Can you work these out from the model? Positions are in its coordinate system, mm. A direction names the side the tool comes from. Give positions to 0.01 mm unless a question says otherwise; leave off trailing zeros. Loops run counter-clockwise (first coordinate to the right, second up) from the corner with the lowest first, then second, coordinate; pieces in that order, holes last. Notation, with made-up numbers: (21, 51.5) - (57, 51.5) arc R33 ccw to (57, 83.5) - close; hole circle Ø4 at (4.25, 76.25). An arc over 180 degrees is marked (long way). Answer in a Markdown table with one row per item.
from build123d import *

# Parameters (mm, degrees)
SKETCH1_R           = 2
BOSS_EXTRUDE1_DEPTH = 75


# Read off the part's stored shape, not the designer's step: M5 Tapped Hole1
with BuildPart() as part:
    # Sketch1 → Boss-Extrude1 (new, symmetric)
    with BuildSketch(Plane(origin=(0, 0, 0), x_dir=(0, 0, -1), z_dir=(1, 0, 0))):
        with BuildLine():
            Line((-10, 0), (-8.2, 0))
            Line((-8.2, 0), (-8.2, -2.5))
            Line((-8.2, -2.5), (-6.43933983, -2.5))
            Line((-6.43933983, -2.5), (-2.839339831, -6.099999999))
            Line((-2.839339831, -6.099999999), (2.839339828, -6.099999999))
            Line((2.839339828, -6.099999999), (6.439339829, -2.499999999))
            Line((6.439339829, -2.499999999), (8.2, -2.499999999))
            Line((8.2, -2.499999999), (8.2, 0))
            Line((8.2, 0), (10, 0))
            Line((10, 0), (10, -5.167329724))
            ThreePointArc((10, -5.167329724), (9.953566515, -5.400766617), (9.821335137, -5.59866486))
            Line((9.821335137, -5.59866486), (8.541421356, -6.87857864))
            ThreePointArc((8.541421356, -6.87857864), (8.323463314, -6.921933191), (8.2, -6.737157284))
            Line((8.2, -6.737157284), (8.2, -3.999999998))
            Line((8.2, -3.999999998), (7.06066017, -3.999999998))
            Line((7.06066017, -3.999999998), (3.9, -7.160660168))
            Line((3.9, -7.160660168), (3.9, -12.83933983))
            Line((3.9, -12.83933983), (6.560660169, -15.499999999))
            Line((6.560660169, -15.499999999), (8.2, -15.499999999))
            Line((8.2, -15.499999999), (8.2, -13.262842712))
            ThreePointArc((8.2, -13.262842712), (8.323463314, -13.078066805), (8.541421356, -13.121421355))
            Line((8.541421356, -13.121421355), (9.821335137, -14.401335136))
            ThreePointArc((9.821335137, -14.401335136), (9.953566515, -14.599233379), (10, -14.832670272))
            Line((10, -14.832670272), (10, -19.499999999))
            ThreePointArc((10, -19.499999999), (9.853553391, -19.85355339), (9.5, -19.999999999))
            Line((9.5, -19.999999999), (4.832670273, -19.999999999))
            ThreePointArc((4.832670273, -19.999999999), (4.599233379, -19.953566514), (4.401335137, -19.821335136))
            Line((4.401335137, -19.821335136), (3.121421356, -18.541421355))
            ThreePointArc((3.121421356, -18.541421355), (3.078066806, -18.323463313), (3.262842712, -18.199999999))
            Line((3.262842712, -18.199999999), (5.5, -18.199999999))
            Line((5.5, -18.199999999), (5.5, -16.560660171))
            Line((5.5, -16.560660171), (2.839339828, -13.899999999))
            Line((2.839339828, -13.899999999), (-2.839339828, -13.899999999))
            Line((-2.839339828, -13.899999999), (-5.5, -16.560660171))
            Line((-5.5, -16.560660171), (-5.5, -18.199999999))
            Line((-5.5, -18.199999999), (-3.262842712, -18.199999999))
            ThreePointArc((-3.262842712, -18.199999999), (-3.078066806, -18.323463313), (-3.121421356, -18.541421355))
            Line((-3.121421356, -18.541421355), (-4.401335137, -19.821335136))
            ThreePointArc((-4.401335137, -19.821335136), (-4.599233379, -19.953566514), (-4.832670273, -19.999999999))
            Line((-4.832670273, -19.999999999), (-9.5, -19.999999999))
            ThreePointArc((-9.5, -19.999999999), (-9.853553391, -19.85355339), (-10, -19.499999999))
            Line((-10, -19.499999999), (-10, -14.832670272))
            ThreePointArc((-10, -14.832670272), (-9.953566515, -14.599233379), (-9.821335137, -14.401335136))
            Line((-9.821335137, -14.401335136), (-8.541421356, -13.121421355))
            ThreePointArc((-8.541421356, -13.121421355), (-8.323463314, -13.078066805), (-8.2, -13.262842712))
            Line((-8.2, -13.262842712), (-8.2, -15.499999999))
            Line((-8.2, -15.499999999), (-6.560660172, -15.499999999))
            Line((-6.560660172, -15.499999999), (-3.9, -12.839339827))
            Line((-3.9, -12.839339827), (-3.9, -7.160660171))
            Line((-3.9, -7.160660171), (-7.06066017, -4.000000001))
            Line((-7.06066017, -4.000000001), (-8.2, -4.000000001))
            Line((-8.2, -4.000000001), (-8.2, -6.737157287))
            ThreePointArc((-8.2, -6.737157287), (-8.323463314, -6.921933193), (-8.541421356, -6.878578643))
            Line((-8.541421356, -6.878578643), (-9.821335137, -5.598664863))
            ThreePointArc((-9.821335137, -5.598664863), (-9.953566515, -5.40076662), (-10, -5.167329726))
            Line((-10, -5.167329726), (-10, 0))
        make_face()
        with Locations((0, -9.999999999)):
            Circle(SKETCH1_R, mode=Mode.SUBTRACT)
    boss_extrude1 = extrude(amount=BOSS_EXTRUDE1_DEPTH, both=True)


with BuildPart() as mirror1_1:
    # Mirror1: Boss-Extrude1 across Top Plane
    add(boss_extrude1.mirror(Plane(origin=(0, 0, 0), x_dir=(1, 0, 0), z_dir=(0, 1, 0))))


with BuildPart() as part_1:
    add(part.part)

    # Mirror1 united with what the copies touc: union Mirror1_1
    add(mirror1_1.part)

    # M5 Tapped Hole1 outline → M5 Tapped Hole1 (revolve, cut)
    with BuildSketch(Plane(origin=(0, 9.999999999, 0), x_dir=(0, 1, 0), z_dir=(0, 0, -1))):
        Polygon((2.1, -62.6), (2, -62.539913938), (2, -75), (2.1, -75), align=None)
        Polygon((2, 75), (2, 62.539913938), (2.1, 62.6), (2.1, 75), align=None)
    revolve(axis=Axis((0, 9.999999999, 0), (1, 0, 0)), mode=Mode.SUBTRACT)

    # M5 Tapped Hole1 2 outline → M5 Tapped Hole1 2 (revolve, cut)
    with BuildSketch(Plane(origin=(0, -9.999999999, 0), x_dir=(0, 1, 0), z_dir=(0, 0, -1))):
        Polygon((2.1, -62.6), (2, -62.539913938), (2, -75), (2.1, -75), align=None)
        Polygon((2, 75), (2, 62.539913938), (2.1, 62.6), (2.1, 75), align=None)
    revolve(axis=Axis((0, -9.999999999, 0), (1, 0, 0)), mode=Mode.SUBTRACT)


solid = part_1.part
Q1. If I drill on line 1 (Y direction, x = 4, z = 0); line 2 (Y direction, x = -60, z = -8.5); line 3 (Z direction, x = -68, y = -10), over which ranges is the centre line in solid material (lowest first)? Write a range as [from, to].
Checked values:
| item | result |
|---|---|
| line 1 | y = [-13.9, -12], [-8, -6.1], [6.1, 8], [12, 13.9] |
| line 2 | y = [-20, -13.09], [-6.91, 6.91], [13.09, 20] |
| line 3 | z = [-3.9, -2.1], [2.1, 3.9] |
Q2. If we mould it in two halves opening along Y, with no side actions, what happens to faces 5 (the face through (1, 17, -10)), 6 (the face through (1, 0, 8.2)), 7 (the face through (1, 10, 3.9)), 8 (the face through (1, 20, 7))? For each: released by +Y, released by -Y, zero draft, split by the parting line, or undercut.
Checked values:
| item | result |
|---|---|
| face 5 | zero draft |
| face 6 | undercut |
| face 7 | undercut |
| face 8 | released by +Y |
Q3. Imagine slicing it at C-C, the plane y = 0. Write out the boundary of the cut face in (x, z).
Checked values:
| item | result |
|---|---|
| outline | (-75, -10) - (75, -10) - (75, -8.2) - (-75, -8.2) - close; (-75, 8.2) - (75, 8.2) - (75, 10) - (-75, 10) - close |
Q4. On a 3-axis mill with a long thin cutter (end or side, diameter ignored), from which of +Z, -Z, +X, -X, +Y, -Y can I reach the whole of each face in a straight line? I mean faces 1 (the face through (1.05, 5.56, -5.5)), 2 (the face through (-68.71, -12.1, 0.09)), 3 (the face through (68.89, 7.9, 0.09)), 4 (the face through (1, 13.9, 0)). Say none if no direction works.
Checked values:
| item | result |
|---|---|
| face 1 | +X, -X |
| face 2 | -X |
| face 3 | +X |
| face 4 | +X, -X, +Y |
Q5. For pin 1 (3.5 mm diameter, centred on y = 10, z = 0, fed in from +X) (1 decimal); pin 2 (1.1 mm diameter, centred on x = -8.5, y = -14, fed in from -Z); pin 3 (3 mm diameter, centred on x = -22.5, y = 10, fed in from +Z); pin 4 (1 mm diameter, centred on x = -7, z = 3, fed in from -Y), each with a flat end and sliding along its axis, tell me the tip position at first contact or that it passes through.
Checked values:
| item | result |
|---|---|
| pin 1 | passes through |
| pin 2 | stops at z = -9.93 |
| pin 3 | stops at z = 3.9 |
| pin 4 | stops at y = -18.92 |
Q6. Imagine slicing it at A-A, the plane y = 10. Write out the boundary of the cut face in (x, z).
Checked values:
| item | result |
|---|---|
| outline | (-75, -3.9) - (75, -3.9) - (75, -2.1) - (62.6, -2.1) - (62.54, -2) - (-62.54, -2) - (-62.6, -2.1) - (-75, -2.1) - close; (-75, 2.1) - (-62.6, 2.1) - (-62.54, 2) - (62.54, 2) - (62.6, 2.1) - (75, 2.1) - (75, 3.9) - (-75, 3.9) - close |
Q7. Imagine slicing it at B-B, the plane z = 0. Count the separate pieces of the cut face and the enclosed holes in it, and give its area (3 significant figures).
Checked values:
| item | result |
|---|---|
| separate pieces | 4 |
| enclosed holes | 0 |
| area | 1,130 mm² |
